Can you work these out from the model? Positions are in its coordinate system, mm. Coordinates: 2 decimals unless noted, no trailing zeros. Order: outer loops, then holes, each group sorted by start corner. A loop starts at its lowest first (then second) coordinate and runs counter-clockwise, first axis right, second up. Notation, with made-up numbers: (22, -24.75) - (63, -24.75) arc R17 cw to (63, 4.25) - close; hole circle Ø5 at (43.25, -1). An arc over 180 degrees is marked (long way). Use a Markdown table: item, result. Add a question column.
(1) If I drill on L1, parallel to Z at x = -1.1, y = -2.5; L2, parallel to Z at x = -0.25, y = -0.25; L3, parallel to Z at x = 0.2, y = 1.75, over which ranges is the centre line in solid material (lowest first)? Write a range as [from, to].
(2) I want a section at C-C (z = -103.5). List the corners of the cut face in (x, y) for me (1 decimal).
(3) I want a section at B-B (x = 0.15). State how many separate pieces and enclosed holes the cut face has, and give its area (3 significant figures).
(4) For pin 1 Ø1 at (x, z) = (0, -68.5) entering from -Y (3 decimals), with a flat end and sliding along its axis, tell me the tip position at first contact or that it passes through.
```python
from build123d import *

# Parameters (mm, degrees)
SKETCH1_R           = 3.175
BOSS_EXTRUDE1_DEPTH = 1.5875
FILLET1_R           = 6.35
CUT_EXTRUDE1_DEPTH  = 0.79375
FILLET2_R           = 2


with BuildPart() as part:
    # Sketch1 → Boss-Extrude1 (new body, symmetric)
    with BuildSketch(Plane(origin=(0, 0, 0), x_dir=(0, 0, -1), z_dir=(1, 0, 0))):
        with BuildLine():
            ThreePointArc((5.499261314, 3.175), (-6.35, 0), (5.499261314, -3.175))
            Line((5.499261314, -3.175), (143.725738686, -3.175))
            ThreePointArc((143.725738686, -3.175), (155.575, 0), (143.725738686, 3.175))
            Line((143.725738686, 3.175), (5.499261314, 3.175))
        make_face()
        Circle(SKETCH1_R, mode=Mode.SUBTRACT)
        with Locations((149.225, 0)):
            Circle(SKETCH1_R, mode=Mode.SUBTRACT)
    extrude(amount=BOSS_EXTRUDE1_DEPTH, both=True)

    # Fillet1
    fillet1_edges = [part.edges().sort_by_distance(p)[0] for p in [
        (0, 3.175, -5.499261314),
        (0, 3.175, -143.725738686),
        (0, -3.175, -143.725738686),
        (0, -3.175, -5.499261314),
    ]]
    fillet(fillet1_edges, radius=FILLET1_R)

    # Sketch2 → Cut-Extrude1 (cut)
    with BuildSketch(Plane.ZY.offset(1.5875)):
        with BuildLine():
            Line((-10.383426303, -3.175), (-8.400260413, -3.175))
            ThreePointArc((-8.400260413, -3.175), (-7.035329576, -3.323430536), (-5.734208949, -3.761783052))
            ThreePointArc((-5.734208949, -3.761783052), (-6.858, 0), (-5.734208949, 3.761783052))
            ThreePointArc((-5.734208949, 3.761783052), (-7.035329576, 3.323430536), (-8.400260413, 3.175))
            Line((-8.400260413, 3.175), (-10.383426303, 3.175))
            ThreePointArc((-10.383426303, 3.175), (-10.858000128, 0), (-10.383426303, -3.175))
        make_face()
    cut_extrude1 = extrude(amount=-CUT_EXTRUDE1_DEPTH, mode=Mode.SUBTRACT)

    # Mirror1: Cut-Extrude1 across plane
    add(cut_extrude1.mirror(Plane.XY.offset(-74.6125)), mode=Mode.SUBTRACT)

    # Fillet2
    fillet2_edges = [part.edges().sort_by_distance(p)[0] for p in [
        (-1.190625, -3.175, -10.383426303),
        (-1.190625, 3.175, -10.383426303),
        (-1.190625, 3.761783052, -5.734208949),
        (-1.190625, -3.761783052, -5.734208949),
        (-1.190625, 3.175, -138.841573697),
        (-1.190625, -3.175, -138.841573697),
        (-1.190625, -3.761783052, -143.490791051),
        (-1.190625, 3.761783052, -143.490791051),
    ]]
    fillet(fillet2_edges, radius=FILLET2_R)


solid = part.part
```
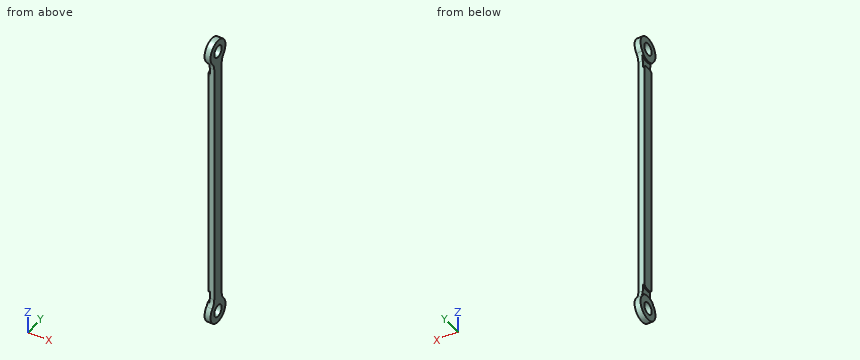
Answers follow:
| question | item | result |
|---|---|---|
| 1 | L1 | z = [-155.06, -151.18], [-147.27, -142.84], [-137.92, -11.31], [-6.39, -1.96], [1.96, 5.84] |
| 1 | L2 | z = [-155.57, -152.39], [-146.06, -3.17], [3.17, 6.35] |
| 1 | L3 | z = [-155.33, -151.87], [-146.58, -2.65], [2.65, 6.1] |
| 2 | outline | (-1.6, -3.2) - (1.6, -3.2) - (1.6, 3.2) - (-1.6, 3.2) - close |
| 3 | separate pieces | 1 |
| 3 | enclosed holes | 2 |
| 3 | area | 1,060 mm² |
| 4 | pin 1 | stops at y = -3.175 |
